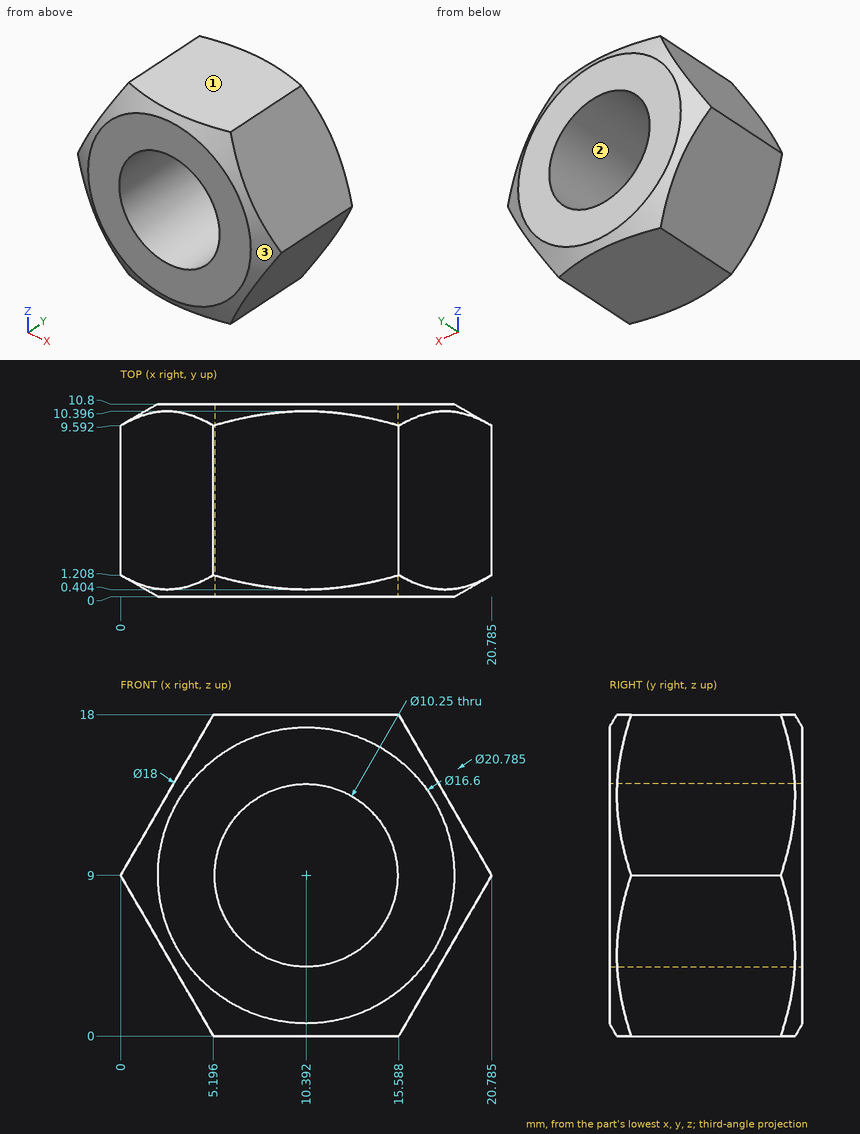
Print and shaded views of the part. All mm, measured from the part's lowest x, y and z. Round coordinates to 2 decimals unless told otherwise and drop trailing zeros. Use a Markdown table: item, result.
1) Flat gauge pin, fed straight in: pin 1 Ø1.5 at (x, y) = (18, 8) entering from -Z. Where does the tip first touch, or does it go through?
Recorded:
| item | result |
|---|---|
| pin 1 | stops at z = 2.88 |
2) Pull direction X, two halves, no side cores. Call the marked faces 1, 2 and 3: pulls with the +X half, pulls with the -X half, needs draft (parallel to the pull), parting line crosses it, or undercut.
Recorded:
| item | result |
|---|---|
| face 1 | needs draft |
| face 2 | undercut |
| face 3 | parting line crosses it |
3) Wall check: L1, parallel to X at y = 9.75, z = 11 (1 decimal); L2, parallel to Z at x = 10, y = 6; L3, parallel to Z at x = 7.75, y = 9.25. Give the ranges that are in metal, low to high.
Recorded:
| item | result |
|---|---|
| L1 | x = 1.2 to 5.7, 15.1 to 19.6 |
| L2 | z = 0 to 3.89, 14.11 to 18 |
| L3 | z = 0 to 4.61, 13.39 to 18 |
